For this review, take the finished solid that the model builds, in its own axes (mm). Face numbers are marked on the shaded views. A direction names the side the tool comes from. Round coordinates to 2 decimals unless told otherwise and drop trailing zeros. Write each loop counter-clockwise with the first axis right and the second up, starting at its lowest first coordinate (ties: lowest second). Pieces come first, ordered by that corner, then holes. Notation, with made-up numbers: (51, -33) -> (72, -33) arc R13 cw to (72, -12) -> close; hole circle Ø2 at (67, 3). An arc over 180 degrees is marked (long way). Answer as CSV lines item,"result". Start each with the question number.
Item 1: Machinability: for the marked faces 1, 2, 3 and 4, which of the approach directions +Z, -Z, +X, -X, +Y, -Y give a long, thin tool a straight path to every point of the face, cutting with its end or side? Answer none if there is none.
Item 2: Wall thickness on probe 1 along Y at (x, z) = (2, 2.25); probe 2 along X at (y, z) = (3.75, 7); probe 3 along Z at (x, y) = (5.75, -0.5): over which ranges is each line inside the solid? List them lowest first. Write a range as from..to.
Item 3: Take a section at A-A on y = 0. Give the boundary of the cut face in (x, z) (3 decimals), then the cut area to 3 significant figures.
Item 4: For pin 1 Ø5 at (x, z) = (19.5, 2) entering from -Y; pin 2 Ø3 at (x, y) = (4.5, -1) entering from +Z; pin 3 Ø1 at (x, y) = (20, 0) entering from +Z, all flat-tipped, find the tip position at first contact; note any pin that passes through.
Item 5: Take a section at B-B on x = 14.25. Give the boundary of the cut face in (y, z).
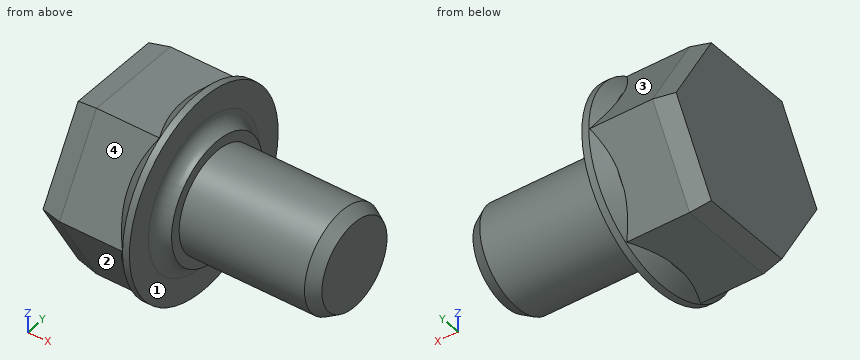
```python
from build123d import *

# Parameters (mm, degrees)
F1_DEPTH = 9
F4_SIZE2 = 2
F4_SIZE  = 0.4
F5_SIZE2 = 0.7
F5_SIZE  = 1.2


with BuildPart() as f1:
    # F0 (on Right) → F1 (new body)
    with BuildSketch(Plane.YZ):
        Polygon((4.8786097747, 8.45), (-4.8786097747, 8.45), (-9.7572195493, 0), (-4.8786097747, -8.45), (4.8786097747, -8.45), (9.7572195493, 0), align=None)
    extrude(amount=F1_DEPTH)

    # F2 (on Front) → F3 (revolve)
    with BuildSketch(Plane.XZ):
        with BuildLine():
            Line((9, 7.315), (9, 0))
            Line((9, 0), (24, 0))
            Line((24, 0), (24, 5))
            Line((24, 5), (10.315, 5))
            Line((10.315, 5), (10.315, 6))
            ThreePointArc((10.315, 6), (9.3851545827, 6.3851545827), (9, 7.315))
        make_face()
        Polygon((7, 8.5), (7, 0), (9, 0), (9, 7.315), (9, 9.815), (8.315, 9.815), align=None)
    revolve(axis=Axis((17.0378703874, 0, 0), (1, 0, 0)))

    # F4
    f4_edges = [f1.edges().sort_by_distance(p)[0] for p in [
        (0, 0, 8.45),
        (0, -7.317915, 4.225),
        (0, -7.317915, -4.225),
        (0, 0, -8.45),
        (0, 7.317915, -4.225),
        (0, 7.317915, 4.225),
    ]]
    f4_side = f1.faces().sort_by_distance((0, 0, 0))[0]
    chamfer(f4_edges, length=F4_SIZE, length2=F4_SIZE2, reference=f4_side)

    # F5
    f5_edges = [f1.edges().sort_by_distance(p)[0] for p in [
        (24, 0, -5),
    ]]
    f5_side = f1.faces().sort_by_distance((17.1575, 0, -5))[0]
    chamfer(f5_edges, length=F5_SIZE, length2=F5_SIZE2, reference=f5_side)


solid = f1.part
```
Output values:
1,face 1,"+X"
1,face 2,"-Z, -X, -Y"
1,face 3,"+Z, -X, +Y"
1,face 4,"+Z, -X, -Y"
2,probe 1,"y = -8.46..8.46"
2,probe 2,"x = 0..9"
2,probe 3,"z = -8.45..8.45"
3,outline,"(0, -8.05) -> (2, -8.45) -> (7, -8.45) -> (7, -8.5) -> (8.315, -9.815) -> (9, -9.815) -> (9, -7.315) arc R1.315 cw to (10.315, -6) -> (10.315, -5) -> (22.8, -5) -> (24, -4.3) -> (24, 4.3) -> (22.8, 5) -> (10.315, 5) -> (10.315, 6) arc R1.315 cw to (9, 7.315) -> (9, 9.815) -> (8.315, 9.815) -> (7, 8.5) -> (7, 8.45) -> (2, 8.45) -> (0, 8.05) -> close"
3,area,"308 mm^2"
4,pin 1,"stops at y = -5"
4,pin 2,"stops at z = 8.45"
4,pin 3,"stops at z = 5"
5,outline,"circle Ø10 at (0, 0)"
